Check sheet for the modelled part. Datum: model origin and axes. Units: mm. Face numbers are marked on the shaded views. A direction names the side the tool comes from. Round coordinates to 2 decimals unless told otherwise and drop trailing zeros.
Item 1: Material ranges on line 1 (Y direction, x = 18, z = 1); line 2 (X direction, y = 15, z = 3.75); line 3 (X direction, y = 16.5, z = 5.75), recorded low to high.
Item 2: Tool access check on the marked faces 4, 5 and 6. Record the directions out of +Z, -Z, +X, -X, +Y, -Y that give a thin tool (end or side, any length) a straight path to the whole face; none if there is none.
Item 3: Release check for a two-part mould opening along Y. For the marked faces 1, 2 and 3 record: +Y half, -Y half, draft (parallel to the pull), parting line (faces both ways), or undercut.
from build123d import *

# Parameters (mm, degrees)
F1_DEPTH = 6.35
F2_COUNT = 13


with BuildPart() as f1:
    # F0 (on Top) → F1 (new body)
    with BuildSketch(Plane.XY):
        with BuildLine():
            ThreePointArc((-2.1437179533, 7.8720496255), (-8.1726662795, 2.7780663468), (-16.0647920269, 2.6720722418))
            ThreePointArc((-16.0647920269, 2.6720722418), (-1.3405858897, -16.2302292777), (16.2855000824, 0))
            ThreePointArc((16.2855000824, 0), (15.6024784663, 4.6669238952), (13.6107061205, 8.9423817764))
            ThreePointArc((13.6107061205, 8.9423817764), (5.9298500897, 5.517014013), (-2.1437179533, 7.8720496255))
        make_face()
        with BuildLine():
            ThreePointArc((-6.7606438886, 14.815910608), (-12.9274256428, 9.9045029751), (-16.0647920269, 2.6720722418))
            ThreePointArc((-16.0647920269, 2.6720722418), (-8.1726662795, 2.7780663468), (-2.1437179533, 7.8720496255))
            ThreePointArc((-2.1437179533, 7.8720496255), (-5.0634420885, 10.9375567243), (-6.7606438886, 14.815910608))
        make_face()
        with BuildLine():
            ThreePointArc((-3.5394354787, 21.5305990191), (-4.554792608, 22.5366665267), (-5.6852551034, 23.4114101898))
            ThreePointArc((-5.6852551034, 23.4114101898), (-7.0109905191, 19.2122527461), (-6.7606438886, 14.815910608))
            ThreePointArc((-6.7606438886, 14.815910608), (-3.8699558436, 15.8190061225), (-0.8426569014, 16.2636847695))
            ThreePointArc((-0.8426569014, 16.2636847695), (-1.8525780021, 19.0704452205), (-3.5394354787, 21.5305990191))
        make_face()
        with BuildLine():
            ThreePointArc((-2.1437179533, 7.8720496255), (5.9298500897, 5.517014013), (13.6107061205, 8.9423817764))
            ThreePointArc((13.6107061205, 8.9423817764), (7.3590855135, 14.5279514502), (-0.8426569014, 16.2636847695))
            ThreePointArc((-0.8426569014, 16.2636847695), (-0.6359958834, 15.0084567204), (-0.5668363347, 13.7382113944))
            ThreePointArc((-0.5668363347, 13.7382113944), (-0.9679319708, 10.7010083415), (-2.1437179533, 7.8720496255))
        make_face()
        with BuildLine():
            ThreePointArc((-0.8426569014, 16.2636847695), (-3.8699558436, 15.8190061225), (-6.7606438886, 14.815910608))
            ThreePointArc((-6.7606438886, 14.815910608), (-5.0634420885, 10.9375567243), (-2.1437179533, 7.8720496255))
            ThreePointArc((-2.1437179533, 7.8720496255), (-0.9679319708, 10.7010083415), (-0.5668363347, 13.7382113944))
            ThreePointArc((-0.5668363347, 13.7382113944), (-0.6359958834, 15.0084567204), (-0.8426569014, 16.2636847695))
        make_face()
    extrude(amount=F1_DEPTH)

    # F2: F1 ×13 about axis
    f2_axis = Axis((0, 0, 6.35), (0, 0, 1))


with BuildPart() as f1_1:
    add(f1.part)
    for i in range(1, F2_COUNT):
        add(f1.part.rotate(f2_axis, i * 360 / F2_COUNT))


solid = f1_1.part
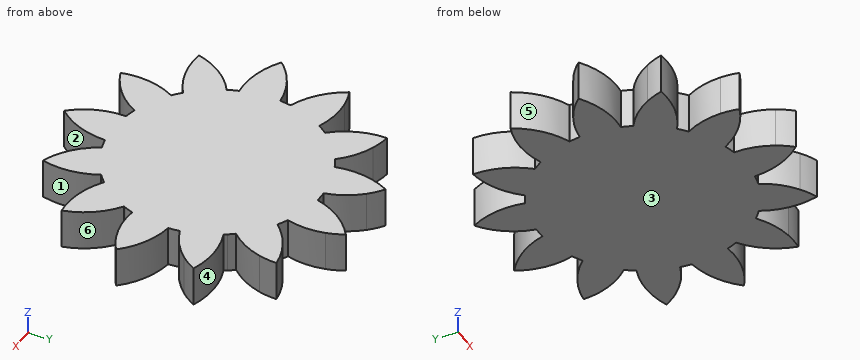
Response values:
1. line 1: y = -13.85 to -9.75, -5.07 to 0.72, 3.7 to 9.27
1. line 2: x = -15.53 to -9.24, -6.8 to 6.87, 9.38 to 15.67
1. line 3: x = -15.82 to -11.23, -7.05 to -0.9, 0.96 to 7.14, 11.49 to 15.95
2. face 4: +Z, -Z
2. face 5: +Z, -Z, -X
2. face 6: +Z, -Z, +X
3. face 1: undercut
3. face 2: -Y half
3. face 3: draft
